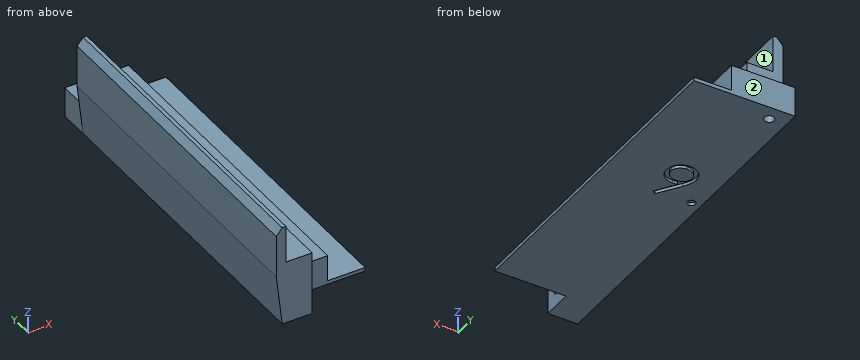
```python
from build123d import *

# Parameters (mm, degrees)
STOCK_GOUX_START         = -23.909074226
STOCK_GOUX_LIKED_1_DEPTH = 47.818148452
SKETCH2_W                = 9.499999796
SKETCH2_H                = 4
CUT_EXTRUDE1_DEPTH       = 126.862368241
SKETCH4_R                = 0.64999997
CUT_EXTRUDE2_DEPTH       = 126.862368241
CIRPATTERN1_COUNT        = 2
CUT_EXTRUDE3_DEPTH       = 0.4
BOSS_EXTRUDE1_DEPTH      = 43.818148451


# Read off the part's stored shape, not the designer's step: Stock-Goux Liked-1
with BuildPart() as part:
    # Stock-Goux Liked-1 outline → Stock-Goux Liked-1 (new body)
    with BuildSketch(Plane(origin=(0, 0, 0), x_dir=(1, 0, 0), z_dir=(0, 1, 0)).offset(STOCK_GOUX_START)):
        Polygon((118.20487789, -113.704878), (118.20487789, -110.204877888), (123.204877796, -110.204877888), (123.204877796, -109.704877872), (109.704877872, -109.704877872), (109.704877872, -123.204877796), (110.204877888, -123.204877796), (110.204877888, -118.20487789), (113.704878, -118.20487789), (113.704878, -113.704878), align=None)
    extrude(amount=STOCK_GOUX_LIKED_1_DEPTH)

    # Sketch2 → Cut-Extrude1 (cut, through all)
    with BuildSketch(Plane.XY.offset(113.704878)):
        with Locations((118.454877898, -21.909074226)):
            Rectangle(SKETCH2_W, SKETCH2_H)
    cut_extrude1 = extrude(amount=-CUT_EXTRUDE1_DEPTH, mode=Mode.SUBTRACT)

    # Sketch4 → Cut-Extrude2 (cut, through all)
    with BuildSketch(Plane(origin=(113.704878, 0, 0), x_dir=(0, 0, -1), z_dir=(1, 0, 0))):
        with Locations((-111.954877944, -21.909074226)):
            Circle(SKETCH4_R)
    cut_extrude2 = extrude(amount=-CUT_EXTRUDE2_DEPTH, mode=Mode.SUBTRACT)

    # CirPattern1: Cut-Extrude1, Cut-Extrude2 ×2 about axis
    cirpattern1_axis = Axis((109.279877871, 0, 109.279877871), (0.7071067811865481, 0, 0.707106781186547))
    add([cut_extrude1.rotate(cirpattern1_axis, i * 360 / CIRPATTERN1_COUNT) for i in range(1, CIRPATTERN1_COUNT)], mode=Mode.SUBTRACT)
    add([cut_extrude2.rotate(cirpattern1_axis, i * 360 / CIRPATTERN1_COUNT) for i in range(1, CIRPATTERN1_COUNT)], mode=Mode.SUBTRACT)

    # Sketch5 → Cut-Extrude3 (cut)
    # profile 1 of 2: a face of its own
    with BuildSketch(Plane(origin=(0, 0, 109.704877872), x_dir=(-1, 0, 0), z_dir=(0, 0, -1))):
        with BuildLine():
            Line((-115.502816358, 2.577164082), (-115.958204979, 2.893900861))
            Line((-115.958204979, 2.893900861), (-114.192620044, 5.474860396))
            add(Edge.make_bspline(
                [(-114.192620044, 5.474860396), (-114.305270378, 5.46108441), (-114.527085168, 5.433958724), (-114.750491053, 5.428975508), (-114.860438553, 5.426523056)],
                knots=[0, 0, 0, 0, 1.015715272, 2, 2, 2, 2], degree=3))
            add(Edge.make_bspline(
                [(-114.860438553, 5.426523056), (-114.927099126, 5.428230438), (-115.057948, 5.431581878), (-115.250319712, 5.458146302), (-115.435169229, 5.499058677), (-115.61200649, 5.560107132), (-115.781496163, 5.635977312), (-115.943268243, 5.730060751), (-116.097104958, 5.840743594), (-116.241354116, 5.967440593), (-116.372548271, 6.106556488), (-116.48943054, 6.253796012), (-116.586569451, 6.410869558), (-116.667262684, 6.574572957), (-116.728459364, 6.747259122), (-116.773022825, 6.926963034), (-116.800459097, 7.114944155), (-116.80372317, 7.242896893), (-116.80538046, 7.3078632)],
                knots=[0, 0, 0, 0, 1.060718605, 2.082097864, 3.085795603, 4.069760067, 5.054557537, 6.03741023, 7.043284206, 8.066802108, 9.088538119, 10.083643548, 11.053783639, 12.022749082, 12.983451788, 13.964007469, 14.966251758, 16, 16, 16, 16], degree=3))
            add(Edge.make_bspline(
                [(-116.80538046, 7.3078632), (-116.8022337, 7.396706327), (-116.796057248, 7.571087363), (-116.746348509, 7.825874344), (-116.66459618, 8.066787073), (-116.550607553, 8.293192139), (-116.407034559, 8.501832709), (-116.234480402, 8.689808329), (-116.033994639, 8.854445421), (-115.810144404, 8.995967104), (-115.568203923, 9.109786313), (-115.314805072, 9.193677615), (-115.051889454, 9.243023915), (-114.873785253, 9.249529692), (-114.784116438, 9.252805107)],
                knots=[0, 0, 0, 0, 1.022988612, 2.007919123, 2.978103895, 3.94594894, 4.918897164, 5.887013414, 6.875921846, 7.89917871, 8.930658928, 9.948724884, 10.967259574, 12, 12, 12, 12], degree=3))
            add(Edge.make_bspline(
                [(-114.784116438, 9.252805107), (-114.696144591, 9.249484669), (-114.522320513, 9.242923795), (-114.266707601, 9.194874308), (-114.021886042, 9.11389063), (-113.789212994, 9.001977207), (-113.573785775, 8.861694989), (-113.380063946, 8.694536639), (-113.212468325, 8.50039804), (-113.07127357, 8.283974636), (-112.957935069, 8.051443113), (-112.876161069, 7.808720854), (-112.825822553, 7.557553459), (-112.819479217, 7.387383485), (-112.816277896, 7.301503024)],
                knots=[0, 0, 0, 0, 1.026385292, 2.028040595, 3.023318987, 4.028184125, 5.03290303, 6.015178782, 7.004435299, 8.016004309, 9.023023918, 10.015172535, 10.998308025, 12, 12, 12, 12], degree=3))
            add(Edge.make_bspline(
                [(-112.816277896, 7.301503024), (-112.818415867, 7.234839332), (-112.822752205, 7.099628708), (-112.853116648, 6.894196515), (-112.904678984, 6.684734999), (-112.96319278, 6.507440104), (-113.019675427, 6.361011916), (-113.072836052, 6.245348335), (-113.131822387, 6.123607472), (-113.200617862, 5.997065873), (-113.274572315, 5.864110417), (-113.358137002, 5.726074632), (-113.449405682, 5.582773288), (-113.514411031, 5.486167857), (-113.547698169, 5.436699338)],
                knots=[0, 0, 0, 0, 1.179839688, 2.393009684, 3.667231171, 4.993948276, 5.694988576, 6.444077775, 7.246288328, 8.089075292, 8.993003841, 9.939041771, 10.944649915, 12, 12, 12, 12], degree=3))
            Line((-113.547698169, 5.436699338), (-115.502816358, 2.577164082))
        make_face()
        with BuildLine():
            add(Edge.make_bspline(
                [(-114.754859627, 6.077805107), (-114.704360773, 6.079184661), (-114.606056671, 6.081870182), (-114.462043571, 6.098215521), (-114.32610966, 6.127196896), (-114.197891822, 6.168779802), (-114.076104442, 6.218956901), (-113.962681961, 6.282841505), (-113.857529453, 6.359071685), (-113.759942786, 6.444724142), (-113.673285243, 6.539884487), (-113.59610003, 6.639483523), (-113.530494429, 6.743958458), (-113.478672484, 6.854617663), (-113.436064754, 6.968767455), (-113.406640647, 7.088246071), (-113.390340499, 7.212431027), (-113.387561785, 7.296792878), (-113.386149691, 7.339664082)],
                knots=[0, 0, 0, 0, 1.163407946, 2.26475976, 3.333800367, 4.359385343, 5.366239384, 6.363380779, 7.350133999, 8.353570782, 9.349036268, 10.310270964, 11.253520213, 12.184142, 13.120487599, 14.056272588, 15.012232024, 16, 16, 16, 16], degree=3))
            add(Edge.make_bspline(
                [(-113.386149691, 7.339664082), (-113.387364662, 7.382553189), (-113.389758912, 7.467071435), (-113.408967299, 7.591440248), (-113.442758775, 7.710626593), (-113.488098654, 7.825282973), (-113.547825371, 7.934467362), (-113.619495981, 8.039550558), (-113.704644854, 8.139866276), (-113.802620939, 8.233055217), (-113.908275056, 8.318957834), (-114.020870535, 8.394769715), (-114.139479312, 8.458308171), (-114.263377772, 8.510739159), (-114.392824062, 8.551654524), (-114.527741583, 8.581077457), (-114.668812105, 8.597354783), (-114.764572438, 8.600115935), (-114.813373249, 8.601523056)],
                knots=[0, 0, 0, 0, 0.972161553, 1.915763587, 2.844109794, 3.775983486, 4.705125789, 5.659731448, 6.655561913, 7.682237399, 8.721216875, 9.739758359, 10.754845918, 11.767244016, 12.7857855, 13.828538656, 14.893392813, 16, 16, 16, 16], degree=3))
            add(Edge.make_bspline(
                [(-114.813373249, 8.601523056), (-114.861749641, 8.600113661), (-114.956663725, 8.597348441), (-115.096480128, 8.581108397), (-115.23048539, 8.551456647), (-115.359556615, 8.510758112), (-115.483451394, 8.45830426), (-115.602054576, 8.394766386), (-115.714676392, 8.318975285), (-115.820229214, 8.232987627), (-115.918378301, 8.14030004), (-116.00206319, 8.039111105), (-116.073897823, 7.934522025), (-116.133542471, 7.825268446), (-116.17890418, 7.71063047), (-116.212689812, 7.591439198), (-116.231899769, 7.467071708), (-116.234293803, 7.382553281), (-116.235508665, 7.339664082)],
                knots=[0, 0, 0, 0, 1.099389452, 2.15699305, 3.192601482, 4.213358962, 5.227959689, 6.245255729, 7.266013209, 8.307253147, 9.336162325, 10.327954924, 11.284637477, 12.215801273, 13.149702402, 14.080068371, 15.025723358, 16, 16, 16, 16], degree=3))
            add(Edge.make_bspline(
                [(-116.235508665, 7.339664082), (-116.234409342, 7.296759493), (-116.232241276, 7.21214379), (-116.211326572, 7.087817334), (-116.176350264, 6.968640183), (-116.129506512, 6.853453528), (-116.067817913, 6.743377443), (-115.992118932, 6.638933801), (-115.903390298, 6.538938627), (-115.802818114, 6.444945542), (-115.692748736, 6.35867231), (-115.575188925, 6.283324331), (-115.452162507, 6.219692896), (-115.323236405, 6.168636385), (-115.189366068, 6.127612367), (-115.04934833, 6.098268935), (-114.903646242, 6.082026965), (-114.804930989, 6.079225895), (-114.754859627, 6.077805107)],
                knots=[0, 0, 0, 0, 0.952633368, 1.87876736, 2.791047057, 3.707742249, 4.635551637, 5.587206343, 6.568248508, 7.601284464, 8.641511608, 9.671105535, 10.699146789, 11.713763218, 12.747829548, 13.806491675, 14.887386225, 16, 16, 16, 16], degree=3))
        make_face(mode=Mode.SUBTRACT)
    # profile 2 of 2: a face of its own
    with BuildSketch(Plane(origin=(0, 0, 109.704877872), x_dir=(-1, 0, 0), z_dir=(0, 0, -1))):
        with BuildLine():
            add(Edge.make_bspline(
                [(-110.984547127, 3.716907671), (-110.949186313, 3.714806426), (-110.879865572, 3.710687181), (-110.779646011, 3.682426644), (-110.688941414, 3.632245931), (-110.608147199, 3.565366319), (-110.541551163, 3.484275616), (-110.489582124, 3.394294467), (-110.461567765, 3.293235864), (-110.457478525, 3.223513453), (-110.45538046, 3.187741005)],
                knots=[0, 0, 0, 0, 1.020151414, 1.999887582, 2.974338812, 3.990962822, 5.007586832, 5.987933904, 6.967670073, 8, 8, 8, 8], degree=3))
            add(Edge.make_bspline(
                [(-110.45538046, 3.187741005), (-110.457549622, 3.152828107), (-110.461827176, 3.083980384), (-110.489517908, 2.983684016), (-110.541947227, 2.893646632), (-110.607687857, 2.81145561), (-110.688961387, 2.744434316), (-110.779860451, 2.694680534), (-110.879630305, 2.664396513), (-110.949147063, 2.660538803), (-110.984547127, 2.658574338)],
                knots=[0, 0, 0, 0, 1.009421747, 1.99056486, 2.972319754, 3.999869655, 5.017953583, 5.993804169, 6.978383603, 8, 8, 8, 8], degree=3))
            add(Edge.make_bspline(
                [(-110.984547127, 2.658574338), (-111.019972699, 2.660467722), (-111.089132694, 2.664164102), (-111.188530141, 2.695302336), (-111.279982784, 2.743967757), (-111.361240489, 2.811580579), (-111.427531716, 2.893223696), (-111.477652054, 2.984304098), (-111.507751324, 3.083693277), (-111.511709865, 3.152771558), (-111.513713794, 3.187741005)],
                knots=[0, 0, 0, 0, 1.022052826, 1.995314843, 2.982371812, 4.00089066, 5.028879526, 6.005146991, 6.990147033, 8, 8, 8, 8], degree=3))
            add(Edge.make_bspline(
                [(-111.513713794, 3.187741005), (-111.511786842, 3.223572022), (-111.508024706, 3.293527686), (-111.477588865, 3.393674638), (-111.427920595, 3.484694521), (-111.360782235, 3.565242602), (-111.280002441, 3.632710994), (-111.188750755, 3.681814262), (-111.088893303, 3.710916152), (-111.019932415, 3.714875861), (-110.984547127, 3.716907671)],
                knots=[0, 0, 0, 0, 1.032775665, 2.016367738, 2.991239715, 4.008302682, 5.025365648, 6.011011707, 6.979408107, 8, 8, 8, 8], degree=3))
        make_face()
    extrude(amount=-CUT_EXTRUDE3_DEPTH, mode=Mode.SUBTRACT)

    # Sketch6 → Boss-Extrude1 (add)
    with BuildSketch(Plane.XZ.offset(23.909074226)):
        Polygon((109.704877872, 109.704877872), (108.911127872, 116.61737789), (108.911127872, 122.258923382), (109.704877872, 123.204877796), align=None)
    extrude(amount=-BOSS_EXTRUDE1_DEPTH)


solid = part.part
```
Geometry check sheet. Reference: the model listing, model coordinates, mm. Face numbers are marked on the shaded views. A direction names the side the tool comes from. Coordinates: 2 decimals unless noted, no trailing zeros. Write each loop counter-clockwise with the first axis right and the second up, starting at its lowest first coordinate (ties: lowest second). Pieces come first, ordered by that corner, then holes. Notation, with made-up numbers: M 24,-25 L 76,-25 A13 ccw 76,-8 Z; hole C 0.25,61.5 d8. An arc over 180 degrees is marked long. One line per item, written item: value. Start each with the question number.
(1) Sectioned sample at B-B, the plane x = 121.75. Enter the section's corners in (y, z).
(2) Sectioned sample at A-A, the plane y = -6.5. Enter the section's corners in (x, z).
(3) Sectioned sample at C-C, the plane z = 117.5. Enter the section's corners in (x, y), and give its area (3 significant figures).
(4) Sectioned sample at D-D, the plane y = 5. Enter the section's corners in (x, z), and give its area (3 significant figures).
(5) Depth check by flat-ended pin: pin 1 (0.6 mm diameter, centred on y = -22, z = 112.5, fed in from +X); pin 2 (1.5 mm diameter, centred on x = 112, y = 12.5, fed in from +Z); pin 3 (1.2 mm diameter, centred on x = 119.5, z = 112, fed in from -Y); pin 4 (1.5 mm diameter, centred on y = -21.91, z = 111.95, fed in from -X). Enter the tip coordinate at first touch or a pass-through.
(6) Tool access check on the marked faces 1 and 2. Record the directions out of +Z, -Z, +X, -X, +Y, -Y that give a thin tool (end or side, any length) a straight path to the whole face; none if there is none.
(7) Scan lines: line 1 along Z through (x, y) = (122, 9); line 2 along Z through (x, y) = (114.75, 12); line 3 along X through (y, z) = (18.5, 121.5). Record each from-to range of solid material in increasing order. Write a range as [from, to].
Filled sheet:
1. outline: M -19.91,109.7 L 23.91,109.7 L 23.91,110.2 L -19.91,110.2 Z
2. outline: M 108.91,116.62 L 109.7,109.7 L 123.2,109.7 L 123.2,110.2 L 118.2,110.2 L 118.2,113.7 L 113.7,113.7 L 113.7,118.2 L 110.2,118.2 L 110.2,123.2 L 109.7,123.2 L 108.91,122.26 Z
3. outline: M 108.91,-23.91 L 113.7,-23.91 L 113.7,19.91 L 108.91,19.91 Z
3. area: 210 mm²
4. outline: M 108.91,116.62 L 109.7,109.7 L 113.85,109.7 L 113.85,110.1 L 114.52,110.1 L 114.52,109.7 L 123.2,109.7 L 123.2,110.2 L 118.2,110.2 L 118.2,113.7 L 113.7,113.7 L 113.7,118.2 L 110.2,118.2 L 110.2,123.2 L 109.7,123.2 L 108.91,122.26 Z
4. area: 64.3 mm²
5. pin 1: x = 113.7
5. pin 2: z = 118.2
5. pin 3: through
5. pin 4: x = 109.36
6. face 1: +Z, +X, +Y, -Y
6. face 2: +Z, -Z, +X, -X, +Y
7. line 1: [109.7, 110.2]
7. line 2: [109.7, 113.7]
7. line 3: [108.91, 110.2]
